from build123d import *

# Parameters (mm, degrees)
F0_W     = 52.736438
F0_H     = 51.140826
F1_DEPTH = 50
F2_R     = 5
F3_DEPTH = 50.001
F4_R     = 5


with BuildPart() as f1:
    # F0 (on Front) → F1 (new body)
    with BuildSketch(Plane.XZ):
        Rectangle(F0_W, F0_H)
    extrude(amount=F1_DEPTH)

    # F2 (on face) → F3 (cut, through all)
    with BuildSketch(Plane.XZ.offset(50)):
        Circle(F2_R)
    extrude(amount=-F3_DEPTH, mode=Mode.SUBTRACT)

    # F4
    f4_edges = [f1.edges().sort_by_distance(p)[0] for p in [
        (-5, -50, 0),
        (-5, 0, 0),
        (26.368219, -25, -25.570413),
        (26.368219, -50, 0),
        (26.368219, 0, 0),
        (26.368219, -25, 25.570413),
        (0, -50, -25.570413),
        (-26.368219, -50, 0),
        (-26.368219, -25, -25.570413),
        (0, 0, -25.570413),
        (0, 0, 25.570413),
        (-26.368219, 0, 0),
        (-26.368219, -25, 25.570413),
    ]]
    fillet(f4_edges, radius=F4_R)


solid = f1.part
Work out the finished part from the listing and answer in its coordinate system (mm). Coordinates: 2 decimals unless noted, no trailing zeros. Write each loop counter-clockwise with the first axis right and the second up, starting at its lowest first coordinate (ties: lowest second). Pieces come first, ordered by that corner, then holes. Notation, with made-up numbers: M -2.5,-10 L 25.5,-10 A6 ccw 25.5,1 Z; hole C 4.25,86.25 d3. An arc over 180 degrees is marked long. Answer as CSV lines item,"result". Start each with the question number.
Item 1: Section C-C on z = 0 is taken. Write down the section's boundary in (x, y).
Item 2: Determine the mould class of faces 1 (the face through (0, -27, 25.57)), 2 (the face through (-1.08, -25.28, -4.88)), 3 (the face through (26.368, -25, 0)) for opening direction Z: released by +Z, released by -Z, zero draft, split by the parting line, or undercut.
Item 3: Section A-A on x = 0 is taken. Write down the section's boundary in (y, z), and give its area (3 significant figures).
Item 4: Section B-B on y = -23 is taken. Write down the section's boundary in (x, z).
Item 5: Consider L1, parallel to Z at x = 0, y = -30; L2, parallel to Y at x = -21.5, z = 6; L3, parallel to X at y = -21, z = -4. Determine where each line is inside the solid, lowest interval first.
Item 6: A flat-ended cylindrical pin translates along its axis: P1, Ø11.5, axis at x = 0, z = 0, coming from the +Y side. Find the tip coordinate at first contact, or state that the pin passes through.
Checks:
1,outline,"M -26.37,-45 A5 ccw -21.37,-50 L -10,-50 A5 ccw -5,-45 L -5,-5 A5 ccw -10,0 L -21.37,0 A5 ccw -26.37,-5 Z; M 5,-45 A5 ccw 10,-50 L 21.37,-50 A5 ccw 26.37,-45 L 26.37,-5 A5 ccw 21.37,0 L 10,0 A5 ccw 5,-5 Z"
2,face 1,"released by +Z"
2,face 2,"undercut"
2,face 3,"zero draft"
3,outline,"M -50,-20.57 A5 ccw -45,-25.57 L -5,-25.57 A5 ccw 0,-20.57 L 0,-10 A5 ccw -5,-5 L -45,-5 A5 ccw -50,-10 Z; M -50,10 A5 ccw -45,5 L -5,5 A5 ccw 0,10 L 0,20.57 A5 ccw -5,25.57 L -50,25.57 Z"
3,area,"2,020 mm²"
4,outline,"M -26.37,-20.57 A5 ccw -21.37,-25.57 L 21.37,-25.57 A5 ccw 26.37,-20.57 L 26.37,20.57 A5 ccw 21.37,25.57 L -21.37,25.57 A5 ccw -26.37,20.57 Z; hole C 0,0 d10"
5,L1,"z = -25.57 to -5, 5 to 25.57"
5,L2,"y = -50 to 0"
5,L3,"x = -26.37 to -3, 3 to 26.37"
6,P1,"stops at y = -2.37"
